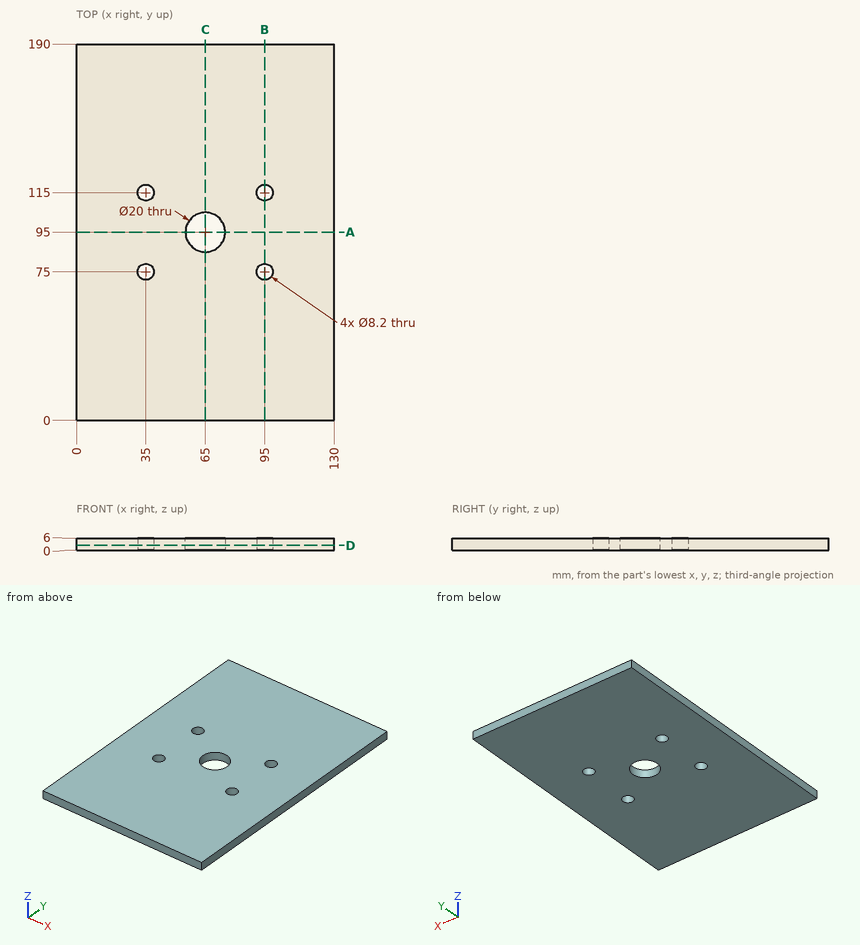
Geometry check sheet. Reference: drawing and pictorial views, mm from the part's lowest x, y, z. Round coordinates to 2 decimals unless told otherwise and drop trailing zeros. Loops run counter-clockwise (first coordinate to the right, second up) from the corner with the lowest first, then second, coordinate; pieces in that order, holes last. Notation, with made-up numbers: (16, -31.75) - (60, -31.75) arc R27 ccw to (60, -6.75) - close; hole circle Ø7 at (48.25, -28.5). An arc over 180 degrees is marked (long way). Answer as CSV lines item,"result".
(1) Cross-section at D-D, the plane z = 2.5. Enter the section's corners in (x, y).
Output values:
outline,"(0, 0) - (130, 0) - (130, 190) - (0, 190) - close; hole circle Ø8.2 at (35, 75); hole circle Ø8.2 at (35, 115); hole circle Ø20 at (65, 95); hole circle Ø8.2 at (95, 75); hole circle Ø8.2 at (95, 115)"
(2) Cross-section at C-C, the plane x = 65. Enter the section's corners in (y, z), and give its area (3 significant figures).
Output values:
outline,"(0, 0) - (85, 0) - (85, 6) - (0, 6) - close; (105, 0) - (190, 0) - (190, 6) - (105, 6) - close"
area,"1,020 mm²"
(3) Cross-section at B-B, the plane x = 95. Enter the section's corners in (y, z).
Output values:
outline,"(0, 0) - (70.9, 0) - (70.9, 6) - (0, 6) - close; (79.1, 0) - (110.9, 0) - (110.9, 6) - (79.1, 6) - close; (119.1, 0) - (190, 0) - (190, 6) - (119.1, 6) - close"
(4) Material ranges on line 1 along Y through (x, z) = (35, 4.2); line 2 along Y through (x, z) = (65, 3.05); line 3 along Y through (x, z) = (96.5, 4.5), recorded low to high.
Output values:
line 1,"y = 0 to 70.9, 79.1 to 110.9, 119.1 to 190"
line 2,"y = 0 to 85, 105 to 190"
line 3,"y = 0 to 71.18, 78.82 to 111.18, 118.82 to 190"
(5) Cross-section at A-A, the plane y = 95. Enter the section's corners in (x, z), and give its area (3 significant figures).
Output values:
outline,"(0, 0) - (55, 0) - (55, 6) - (0, 6) - close; (75, 0) - (130, 0) - (130, 6) - (75, 6) - close"
area,"660 mm²"
